CAD build for the part. Positions are in the model's coordinates, mm. Coordinates: 2 decimals unless noted, no trailing zeros. Order: outer loops, then holes, each group sorted by start corner. A loop starts at its lowest first (then second) coordinate and runs counter-clockwise, first axis right, second up. Notation, with made-up numbers: M -22,49 L 33,49 A22 ccw 33,82 Z; hole C 61.25,-32 d4. An arc over 180 degrees is marked long. One line per item, written item: value.
from build123d import *

# Parameters (mm, degrees)
F0_R     = 290
F1_DEPTH = 950
F2_T     = -7.62
F3_R     = 10


with BuildPart() as f1:
    # F0 (on Top) → F1 (new body)
    with BuildSketch(Plane.XY):
        Circle(F0_R)
    extrude(amount=-F1_DEPTH)

    # F2
    f2_openings = [f1.faces().sort_by_distance(p)[0] for p in [
        (0, 0, 0),
    ]]
    offset(amount=F2_T, openings=f2_openings)

    # F3
    f3_edges = [f1.edges().sort_by_distance(p)[0] for p in [
        (-290, 0, -950),
    ]]
    fillet(f3_edges, radius=F3_R)


solid = f1.part
Q1. Drill centre lines: line 1 along Y through (x, z) = (0, -380.5); line 2 along Z through (x, y) = (-185.5, 111.5); line 3 along X through (y, z) = (225.5, -285). Where is each one in solid material? Low to high.
Recorded:
line 1: y = -290 to -282.38, 282.38 to 290
line 2: z = -950 to -942.38
line 3: x = -182.35 to -169.97, 169.97 to 182.35
Q2. Pin check, flat tips, straight feed: pin 1 Ø1.5 at (x, y) = (-174, 109.5) entering from +Z; pin 2 Ø1 at (x, z) = (198.5, -448) entering from +Y; pin 3 Ø10 at (x, z) = (-121.5, -657) entering from +Y; pin 4 Ø10 at (y, z) = (3, -437) entering from +X. Stop position of each tip, or through.
Recorded:
pin 1: stops at z = -942.38
pin 2: stops at y = 211.89
pin 3: stops at y = 265.57
pin 4: stops at x = 290
Q3. Slice it at A-A (x = 0). List the corners of the cut face in (y, z).
Recorded:
outline: M -290,-940 A10 ccw -280,-950 L 280,-950 A10 ccw 290,-940 L 290,0 L 282.38,0 L 282.38,-942.38 L -282.38,-942.38 L -282.38,0 L -290,0 Z
Q4. Mould opens along X. For faces 1 (the face through (63, -278, 0)), 2 (the face through (276.608, 87.108, -463.42)), 3 (the face through (-61.214, -275.665, -464.593)), 4 (the face through (-4, 4, -942.38)) say: released by +X, released by -X, zero draft, split by the parting line, or undercut.
Recorded:
face 1: zero draft
face 2: split by the parting line
face 3: undercut
face 4: undercut
Q5. Slice it at C-C (z = -660.5). List the corners of the cut face in (x, y), plus the area to 3 significant figures.
Recorded:
outline: C 0,0 d580; hole C 0,0 d564.76
area: 13,700 mm^2
